Autodesk Inventor part; units mm, degrees
ref_plane "YZ Plane" through (0, 0, 0) normal (1, 0, 0) x (0, 1, 0)
ref_plane "XZ Plane" through (0, 0, 0) normal (0, 1, 0) x (-1, 0, 0)
ref_plane "XY Plane" through (0, 0, 0) normal (0, 0, 1) x (1, 0, 0)
sketch "roof_sketch" plane through (0, 0, 0) normal (0, 0, 1) x (1, 0, 0)
  line L0 (-26.6, 0) -> (26.6, 0) construction
  line L1 (0, -3.8) -> (0, 22.8) construction
  line L2 (-16, 0) -> (16, 0)
  line L3 (-19, 0) -> (-16, 0)
  line L4 (16, 0) -> (19, 0)
  arc A0 (16, 0) -> (-16, 0) centre (0, 0) ccw
  arc A1 (19, 0) -> (-19, 0) centre (0, 0) ccw
  line L5 (-19, 0) -> (-16, 0)
  line L6 (16, 0) -> (19, 0)
  dimension "d1" = 32
  dimension "d5" = 0
  dimension "d6" = 3
extrude "roof" add sketch "roof_sketch" along normal blind 126.5 contours L3 A1 L4 A0
sketch "bolt_sketch" plane through (16, 0, 0) normal (0, -1, 0) x (1, 0, 0)
  line L0 (-52.4, 0) -> (20.4, 0) construction
  line L1 (-16, -25.3) -> (-16, 151.8) construction
  line L2 (3, 0) -> (3, 126.5)
  line L3 (3, 41.5) -> (10, 41.5)
  line L4 (10, 41.5) -> (10, 0)
  line L5 (10, 0) -> (3, 0)
  line L6 (3, 0) -> (3, 41.5)
  circle A0 centre (6.5, 31.5) radius 1.5
  circle A1 centre (6.5, 11.5) radius 1.5
  line L7 (-35, 41.5) -> (-42, 41.5)
  line L8 (-42, 41.5) -> (-42, 0)
  line L9 (-42, 0) -> (-35, 0)
  line L10 (-35, 0) -> (-35, 41.5)
  circle A2 centre (-38.5, 31.5) radius 1.5
  circle A3 centre (-38.5, 11.5) radius 1.5
  point P0 (-16, 0)
  dimension "d9" = 41.5
  dimension "d10" = 3
  dimension "d11" = 3
  dimension "d12" = 10
  dimension "d13" = 20
  dimension "d14" = 7
  dimension "d16" = 3.5
  dimension "d17" = 3.5
extrude "bolt_opposite" add sketch "bolt_sketch" against normal blind 1.5
sketch "error1_" plane through (-19, 0, 0) normal (1, 0, 0) x (0, 0, -1)
  line L0 (0, 1.5) -> (-41.5, 1.5)
  line L1 (0, 0) -> (0, 1.5)
  line L2 (-41.5, 0) -> (0, 0)
  line L3 (-41.5, 0) -> (-41.5, 1.5)
extrude "error1" add sketch "error1_" along normal blind 1.5
sketch "error2_" plane through (19, 0, 0) normal (-1, 0, 0) x (0, 0, 1)
  line L0 (0, 0) -> (0, 1.5)
  line L1 (0, 1.5) -> (41.5, 1.5)
  line L2 (41.5, 0) -> (0, 0)
  line L3 (41.5, 0) -> (41.5, 1.5)
extrude "error2" add sketch "error2_" along normal blind 1.5
ref_plane "for_button" through (16, 19, 126.5) normal (0, -1, 0) x (1, 0, 0)
sketch "button_sketch" plane through (16, 19, 126.5) normal (0, -1, 0) x (1, 0, 0)
  line L0 (-13, -25) -> (-19, -25)
  line L1 (-19, -25) -> (-19, -40)
  line L2 (-19, -40) -> (-13, -40)
  line L3 (-13, -40) -> (-13, -25)
  line L4 (-35, -85) -> (-35, 0)
  line L5 (3, 0) -> (-35, 0)
  circle A0 centre (-15.9407, -106.5001) radius 1.5
  circle A1 centre (-15.9407, -116.5) radius 1.5
  line L6 (2.9407, -126.5) -> (-34.9407, -126.5)
  line L7 (-34.9407, -126.5) -> (-34.9407, -85)
  point P0 (-16, -126.5)
  dimension "d25" = 6
  dimension "d26" = 15
  dimension "d27" = 16
  dimension "d28" = 25
  dimension "d43" = 3
  dimension "d44" = 3
  dimension "d45" = 10
  dimension "d46" = 20
  dimension "d47" = 19
  dimension "d48" = 19
extrude "button" cut sketch "button_sketch" along normal blind 10 contours L3 L2 L1 L0
fillet "so_hurt" radius 0.7 4 edges at (26, 1.5, 20.75) (22.4703, 1.5, 41.5) (-26, 1.5, 20.75) (-22.4703, 1.5, 41.5)
extrude "bar" cut sketch "button_sketch" along normal blind 10 contours A0 | A1
equation "\"d11\" = d10"
equation "\"d16\" = 0.5 * d14"
equation "\"d17\" = d16"
equation "\"d44\" = d43"
equation "\"d48\" = d47"
properties part number "smart_pen4"
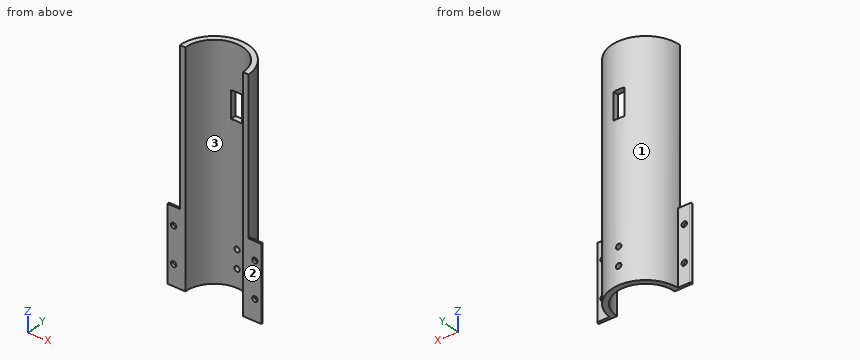
Can you work these out from the model? Positions are in its coordinate system, mm. Face numbers are marked on the shaded views. Give positions to 0.01 mm unless a question says otherwise; leave off trailing zeros. Loops run counter-clockwise (first coordinate to the right, second up) from the corner with the lowest first, then second, coordinate; pieces in that order, holes last. Notation, with made-up numbers: (-22, -13) -> (1, -13) arc R22 ccw to (1, 25) -> close; hole circle Ø7 at (18.25, 5). An arc over 180 degrees is marked (long way). Write item = value, one per line.
1) Suppose I cut it at B-B on z = 31.5. Write out the boundary of the cut face in (x, y).
Check result:
outline = (-26, 0) -> (-24, 0) -> (-24, 1.5) -> (-25.3, 1.5) arc R0.7 ccw to (-26, 0.8) -> close; (-21, 0) -> (-16, 0) arc R16 cw to (16, 0) -> (21, 0) -> (21, 1.5) -> (18.94, 1.5) arc R19 ccw to (-18.94, 1.5) -> (-21, 1.5) -> close; (24, 0) -> (26, 0) -> (26, 0.8) arc R0.7 ccw to (25.3, 1.5) -> (24, 1.5) -> close
2) I need wall thicknesses on L1, parallel to Z at x = -22.5, y = 0.5; L2, parallel to X at y = 14.5, z = 87; L3, parallel to X at y = 1, z = 59.5. Which ranges of each line are inside material? Lowest first, please. Write a range as from..to.
Check result:
L1 = 0..10, 13..30, 33..41.5
L2 = -12.28..-6.76, 6.76..12.28
L3 = -18.97..-15.97, 15.97..18.97
3) Suppose I cut it at D-D on y = 11.75. Write out the boundary of the cut face in (x, z).
Check result:
outline = (-14.93, 0) -> (-10.86, 0) -> (-10.86, 126.5) -> (-14.93, 126.5) -> close; (10.86, 0) -> (14.93, 0) -> (14.93, 126.5) -> (10.86, 126.5) -> close
4) Will these pins go through, and if not, where does the flat tip stop? pin 1 (12 mm diameter, centred on x = 7.5, z = 71, fed in from -Y); pin 2 (1.9 mm diameter, centred on x = -21, z = 24, fed in from +Y); pin 3 (4 mm diameter, centred on x = -10.5, y = 8.5, fed in from -Z); pin 4 (3.5 mm diameter, centred on y = 17.5, z = 96.5, fed in from -X).
Check result:
pin_1 = 8.59
pin_2 = 1.5
pin_3 = through
pin_4 = -10.63
5) Suppose I cut it at A-A on z = 96. Write out the boundary of the cut face in (x, y).
Check result:
outline = (-19, 0) -> (-16, 0) arc R16 cw to (-3, 15.72) -> (-3, 18.76) arc R19 ccw to start; (3, 15.72) arc R16 cw to (16, 0) -> (19, 0) arc R19 ccw to (3, 18.76) -> close
6) Suppose I cut it at C-C on x = 22.5. Write out the boundary of the cut face in (y, z).
Check result:
outline = (0, 0) -> (1.5, 0) -> (1.5, 10) -> (0, 10) -> close; (0, 13) -> (1.5, 13) -> (1.5, 30) -> (0, 30) -> close; (0, 33) -> (1.5, 33) -> (1.5, 40.8) arc R0.7 ccw to (0.8, 41.5) -> (0, 41.5) -> close
7) Thinking about a two-plate mould opening in X: for the marked faces 1, 2 and 3, which applies, released by +X, released by -X, zero draft, split by the parting line, or undercut?
Check result:
face_1 = split by the parting line
face_2 = zero draft
face_3 = undercut
